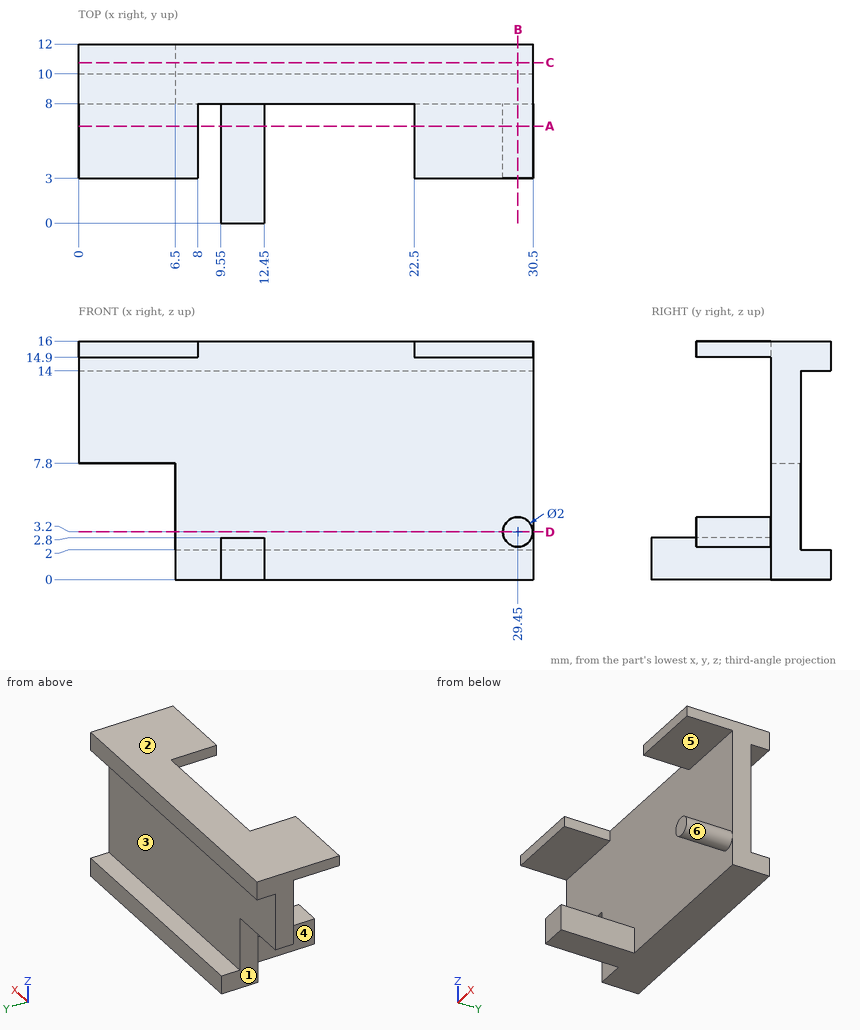
Input: dimensioned drawing with shaded views. Units: mm. Origin: part minimum x, y, z. A direction names the side the tool comes from. Round coordinates to 2 decimals unless told otherwise and drop trailing zeros. Loops run counter-clockwise (first coordinate to the right, second up) from the corner with the lowest first, then second, coordinate; pieces in that order, holes last. Notation, with made-up numbers: (80, 3) -> (93, 3) arc R11 ccw to (93, 8) -> close; hole circle Ø5 at (68, 66). An arc over 180 degrees is marked (long way). Use one line per item in the form item = value. Start each with the question number.
1) Section A-A on y = 6.5. Output: boundary loops of the cut face in (x, z), then the cut area to 3 significant figures.
2) Section B-B on x = 29.45. Output: boundary loops of the cut face in (y, z).
3) Draft query along Z for the marked faces 1, 2 and 3. Return one class per face: released by +Z, released by -Z, zero draft, split by the parting line, or undercut.
4) Section C-C on y = 10.75. Output: boundary loops of the cut face in (x, z), then the cut area to 3 significant figures.
5) Line query: L1, parallel to Z at x = 6, y = 3.75; L2, parallel to Y at x = 17.5, z = 8.5; L3, parallel to X at y = 4.25, z = 1. Output: solid intervals per line, ascending.
6) Access query for the marked faces 4, 5 and 6. Directions: +Z, -Z, +X, -X, +Y, -Y. A direction counts if a zero-diameter tool reaches every point of the face in a straight line with its end or side. Return the directions, or none.
7) First-contact query: P1, Ø3, axis at x = 15.5, y = 7.5, coming from the +Z side; P2, Ø1.5, axis at x = 5.5, y = 5.5, coming from the -Z side; P3, Ø2, axis at y = 3.5, z = 4.5, coming from the +X side; P4, Ø0.6, axis at x = 30, z = 3.5, coming from the -Y side. Flat tips, straight axial feed; report the tip coordinate or a pass-through.
8) Section D-D on z = 3.2. Output: boundary loops of the cut face in (x, y), then the cut area to 3 significant figures.
Response:
q1.outline = (0, 14.9) -> (8, 14.9) -> (8, 16) -> (0, 16) -> close; (9.55, 0) -> (12.45, 0) -> (12.45, 2.8) -> (9.55, 2.8) -> close; (22.5, 14.9) -> (30.5, 14.9) -> (30.5, 16) -> (22.5, 16) -> close; circle Ø2 at (29.45, 3.2)
q1.area = 28.9 mm^2
q2.outline = (3, 2.2) -> (8, 2.2) -> (8, 0) -> (12, 0) -> (12, 2) -> (10, 2) -> (10, 14) -> (12, 14) -> (12, 16) -> (3, 16) -> (3, 14.9) -> (8, 14.9) -> (8, 4.2) -> (3, 4.2) -> close
q3.face_1 = zero draft
q3.face_2 = released by +Z
q3.face_3 = undercut
q4.outline = (0, 14) -> (30.5, 14) -> (30.5, 16) -> (0, 16) -> close; (6.5, 0) -> (30.5, 0) -> (30.5, 2) -> (6.5, 2) -> close
q4.area = 109 mm^2
q5.L1 = 14.9 to 16
q5.L2 = 8 to 10
q5.L3 = 9.55 to 12.45
q6.face_4 = +Z, -Z, -X, -Y
q6.face_5 = +X, -X, -Y
q6.face_6 = -Y
q7.P1 = 16
q7.P2 = 14.9
q7.P3 = 30.4
q7.P4 = 3
q8.outline = (6.5, 8) -> (28.45, 8) -> (28.45, 3) -> (30.45, 3) -> (30.45, 8) -> (30.5, 8) -> (30.5, 10) -> (6.5, 10) -> close
q8.area = 58.0 mm^2
